from build123d import *

# Parameters (mm, degrees)
SKETCH1_R           = 20
SKETCH1_R_2         = 2.5
BOSS_EXTRUDE1_DEPTH = 8
SKETCH2_W           = 3
SKETCH2_H           = 3
BOSS_EXTRUDE2_DEPTH = 10
SKETCH3_R           = 7.5
BOSS_EXTRUDE3_DEPTH = 25
SKETCH4_R           = 10
BOSS_EXTRUDE4_DEPTH = 5


with BuildPart() as part:
    # Sketch1 → Boss-Extrude1 (new body)
    with BuildSketch(Plane.XY):
        Circle(SKETCH1_R)
        with Locations((3.80920927, 14.508270908)):
            Circle(SKETCH1_R_2, mode=Mode.SUBTRACT)
        with Locations((14.397906738, 4.207528657)):
            Circle(SKETCH1_R_2, mode=Mode.SUBTRACT)
        with Locations((11.022029668, -10.174031029)):
            Circle(SKETCH1_R_2, mode=Mode.SUBTRACT)
        with Locations((-3.044078256, -14.687390408)):
            Circle(SKETCH1_R_2, mode=Mode.SUBTRACT)
        with Locations((-14.157363478, -4.954934573)):
            Circle(SKETCH1_R_2, mode=Mode.SUBTRACT)
        with Locations((-11.538785608, 9.58359544)):
            Circle(SKETCH1_R_2, mode=Mode.SUBTRACT)
    extrude(amount=BOSS_EXTRUDE1_DEPTH)

    # Sketch2 → Boss-Extrude2 (add)
    with BuildSketch(Plane.XY.offset(8)):
        Rectangle(SKETCH2_W, SKETCH2_H)
    extrude(amount=BOSS_EXTRUDE2_DEPTH)

    # Sketch3 → Boss-Extrude3 (add)
    with BuildSketch(Plane(origin=(0, 0, 0), x_dir=(-1, 0, 0), z_dir=(0, 0, -1))):
        with Locations(Location((0, 0, 0), (0, 0, 180))):
            Circle(SKETCH3_R)
    extrude(amount=BOSS_EXTRUDE3_DEPTH)

    # Sketch4 → Boss-Extrude4 (add)
    with BuildSketch(Plane(origin=(0, 0, 0), x_dir=(-1, 0, 0), z_dir=(0, 0, -1))):
        with Locations(Location((0, 0, 0), (0, 0, 180))):
            Circle(SKETCH4_R)
    extrude(amount=BOSS_EXTRUDE4_DEPTH)


solid = part.part
The listing builds one solid part. Answer for the finished solid, in the listing's coordinates (mm). A direction names the side the tool comes from. Round coordinates to 2 decimals unless told otherwise and drop trailing zeros. Order: outer loops, then holes, each group sorted by start corner. A loop starts at its lowest first (then second) coordinate and runs counter-clockwise, first axis right, second up. Notation, with made-up numbers: (60.5, -19.5) -> (73.5, -19.5) arc R18 ccw to (73.5, -6.5) -> close; hole circle Ø2 at (59.25, -31.5). An arc over 180 degrees is marked (long way). Write each question's results on one line, items separated by ' | '. Start each with the question number.
Q1. Find section A-A (y = 13). Determine the outline of the cut face in (x, z), then the cut area to 3 significant figures.
Q2. Straight lines are drawn through the part: probe 1 along Z at (x, y) = (6, -11); probe 2 along Z at (x, y) = (-3.5, 4); probe 3 along X at (y, z) = (-15.5, 5). For each, find the intervals that lie inside material, in ascending order. Write a range as from..to.
Q3. Find section D-D (z = 10.5). Determine the outline of the cut face in (x, y).
Q4. The mould has two halves that part along Y. Classify faces 6 (the cylindrical face through (4.032, -6.324, -14.86)), 7 (the flat face through (1.5, 0, 13)), 8 (the cylindrical face through (-16, -3.265, 3.944)), 9 (the cylindrical face through (10.697, -7.695, 3.944)): pulls with the +Y half, pulls with the -Y half, needs draft (parallel to the pull), parting line crosses it, or undercut.
Q5. Find section B-B (x = -2.5). Determine the outline of the cut face in (y, z), then the cut area to 3 significant figures.
Q6. Which of the six approach directions +Z, -Z, +X, -X, +Y, -Y give full straight-line access (tool end or side, diameter ignored) to faces 1 (the cylindrical face through (-3.586, -17.128, 3.944)), 2 (the flat face through (-1.5, 0, 13)), 3 (the flat face through (0, -1.5, 13)), 4 (the flat face through (-5, 9, 0)), 5 (the flat face through (0, 1.5, 13))?
Q7. Find section C-C (y = -14). Determine the outline of the cut face in (x, z).
Q8. Each of these flat-tipped pins is pushed along its axis until it touches: pin 1 (6.5 mm diameter, centred on x = -14.16, y = -4.95, fed in from +Z); pin 2 (10 mm diameter, centred on y = -6, z = 12, fed in from -X); pin 3 (4.5 mm diameter, centred on x = 14.4, y = 4.21, fed in from +Z); pin 4 (2 mm diameter, centred on x = 7.5, z = -2.5, fed in from +Y). Where does it stop, or does it pass through?
Worked answers:
1) outline: (-15.2, 0) -> (1.82, 0) -> (1.82, 8) -> (-15.2, 8) -> close; (5.8, 0) -> (15.2, 0) -> (15.2, 8) -> (5.8, 8) -> close | area: 211 mm2
2) probe 1: z = 0..8 | probe 2: z = -25..8 | probe 3: x = -12.64..-5.41, -0.68..12.64
3) outline: (-1.5, -1.5) -> (1.5, -1.5) -> (1.5, 1.5) -> (-1.5, 1.5) -> close
4) face 6: parting line crosses it | face 7: needs draft | face 8: undercut | face 9: undercut
5) outline: (-19.84, 0) -> (-17.13, 0) -> (-17.13, 8) -> (-19.84, 8) -> close; (-12.25, 0) -> (-9.68, 0) -> (-9.68, -5) -> (-7.07, -5) -> (-7.07, -25) -> (7.07, -25) -> (7.07, -5) -> (9.68, -5) -> (9.68, 0) -> (19.84, 0) -> (19.84, 8) -> (-12.25, 8) -> close | area: 658 mm2
6) face 1: +Z, -Z | face 2: +Z, -X, +Y, -Y | face 3: +Z, +X, -X, -Y | face 4: -Z | face 5: +Z, +X, -X, +Y
7) outline: (-14.28, 0) -> (-5.45, 0) -> (-5.45, 8) -> (-14.28, 8) -> close; (-0.64, 0) -> (14.28, 0) -> (14.28, 8) -> (-0.64, 8) -> close
8) pin 1: stops at z = 8 | pin 2: stops at x = -19.77 | pin 3: passes through | pin 4: stops at y = 7.6
